```python
from build123d import *

# Parameters (mm, degrees)
SKETCH1_W               = 203.2
SKETCH1_H               = 15.875
BOSS_EXTRUDE1_DEPTH     = 1.524
BOSS_EXTRUDE2_START     = -15.875
BOSS_EXTRUDE2_OUTLINE_R = 2.413
BOSS_EXTRUDE2_DEPTH     = 15.875


# Read off the part's stored shape, not the designer's step: Boss-Extrude2
with BuildPart() as part:
    # Sketch1 → Boss-Extrude1 (new body)
    with BuildSketch(Plane(origin=(0, 0, 0), x_dir=(1, 0, 0), z_dir=(0, 1, 0))):
        Rectangle(SKETCH1_W, SKETCH1_H)
    extrude(amount=BOSS_EXTRUDE1_DEPTH)

    # Boss-Extrude2 outline → Boss-Extrude2 (add)
    with BuildSketch(Plane.XY.offset(7.9375).offset(BOSS_EXTRUDE2_START)):
        with BuildLine():
            add(Edge.make_bspline(
                [(107.228546138, 6.692607406), (106.366027923, 7.18125968), (105.140033894, 7.42790314), (103.583408394, 7.287922485), (101.756786703, 6.577932625), (99.786331846, 5.041015057)],
                knots=[0, 0, 0, 0, 0, 0, 1, 1, 1, 1, 1, 1], degree=5))
            ThreePointArc((107.228546138, 6.692607406), (108.258782429, 4.761783473), (107.30453503, 2.792296286))
            add(Edge.make_bspline(
                [(101.6, 1.524), (103.258114517, 1.448306251), (104.638933259, 1.583946831), (105.766741539, 1.881154947), (106.652889556, 2.297992507), (107.30453503, 2.792296286)],
                knots=[0, 0, 0, 0, 0, 0, 1, 1, 1, 1, 1, 1], degree=5))
            Line((101.6, 1.524), (101.6, 0))
            add(Edge.make_bspline(
                [(101.6, 0), (104.748480566, -0.003746591), (109.050367624, 0.259943099), (110.73800353, 3.235869603), (109.946934459, 5.044027479), (108.94689031, 7.25796652)],
                knots=[0, 0, 0, 0, 0, 0, 1, 1, 1, 1, 1, 1], degree=5))
            add(Edge.make_bspline(
                [(108.94689031, 7.25796652), (106.455515071, 10.263008134), (101.235622898, 14.016404122), (98.534099755, 12.238404022), (96.99562172, 12.065011937)],
                knots=[0, 0, 0, 0, 0, 1, 1, 1, 1, 1], degree=4))
            ThreePointArc((96.99562172, 12.065011937), (93.706192437, 6.691697876), (99.786331846, 5.041015057))
        make_face()
        with Locations((97.364988112, 8.145377073)):
            Circle(BOSS_EXTRUDE2_OUTLINE_R, mode=Mode.SUBTRACT)
    extrude(amount=BOSS_EXTRUDE2_DEPTH)


solid = part.part
```
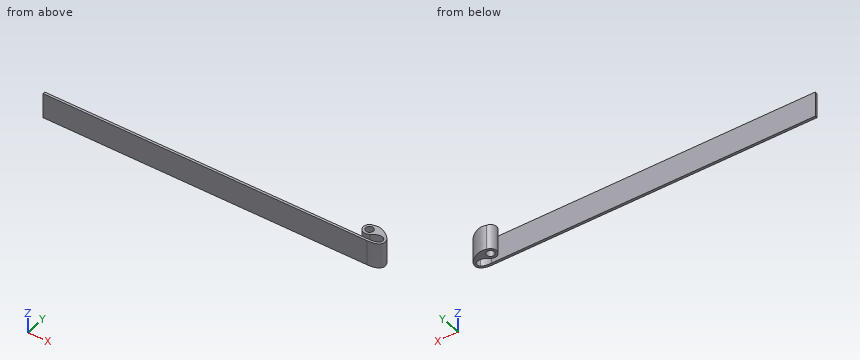
Input: part model. Units: mm. Frame: model coordinates. Give positions to 0.01 mm unless a question says otherwise; leave off trailing zeros. Write each loop counter-clockwise with the first axis right and the second up, starting at its lowest first coordinate (ties: lowest second). Pieces come first, ordered by that corner, then holes. Notation, with made-up numbers: (-21, 17.25) - (9, 17.25) arc R27 cw to (9, 39.25) - close; hole circle Ø11 at (-32.75, 89.25). An arc over 180 degrees is marked (long way). Write item = value, one per line. Start each with the question number.
1. First-contact query: pin 1 Ø4.5 at (x, y) = (97.36, 8.15) entering from -Z; pin 2 Ø1 at (y, z) = (7.5, -2.5) entering from -X; pin 3 Ø8 at (x, z) = (-2.5, 0) entering from +Y. Flat tips, straight axial feed; report the tip coordinate or a pass-through.
2. Ray query, L1, parallel to Y at x = 3, z = 2.75; L2, parallel to X at y = 6.5, z = -0.25; L3, parallel to Y at x = 95.5, z = 6.5. Return the intervals inside material, ascending.
3. Section query A-A, the plane x = -82.5. Output: boundary loops of the cut face in (y, z).
Check sheet entries:
q1.pin_1 = through
q1.pin_2 = 93.43
q1.pin_3 = 1.52
q2.L1 = 0 to 1.52
q2.L2 = 93.79 to 95.6, 99.13 to 102.18, 107.47 to 109.28
q2.L3 = 0 to 1.52, 4.68 to 6.61, 9.68 to 11.61
q3.outline = (0, -7.94) - (1.52, -7.94) - (1.52, 7.94) - (0, 7.94) - close
